Could you check a few things on this drawing? It's one solid part, dimensions in mm from its lowest x, y, z. A direction names the side the tool comes from. Round coordinates to 2 decimals unless told otherwise and drop trailing zeros. Loops run counter-clockwise (first coordinate to the right, second up) from the corner with the lowest first, then second, coordinate; pieces in that order, holes last.
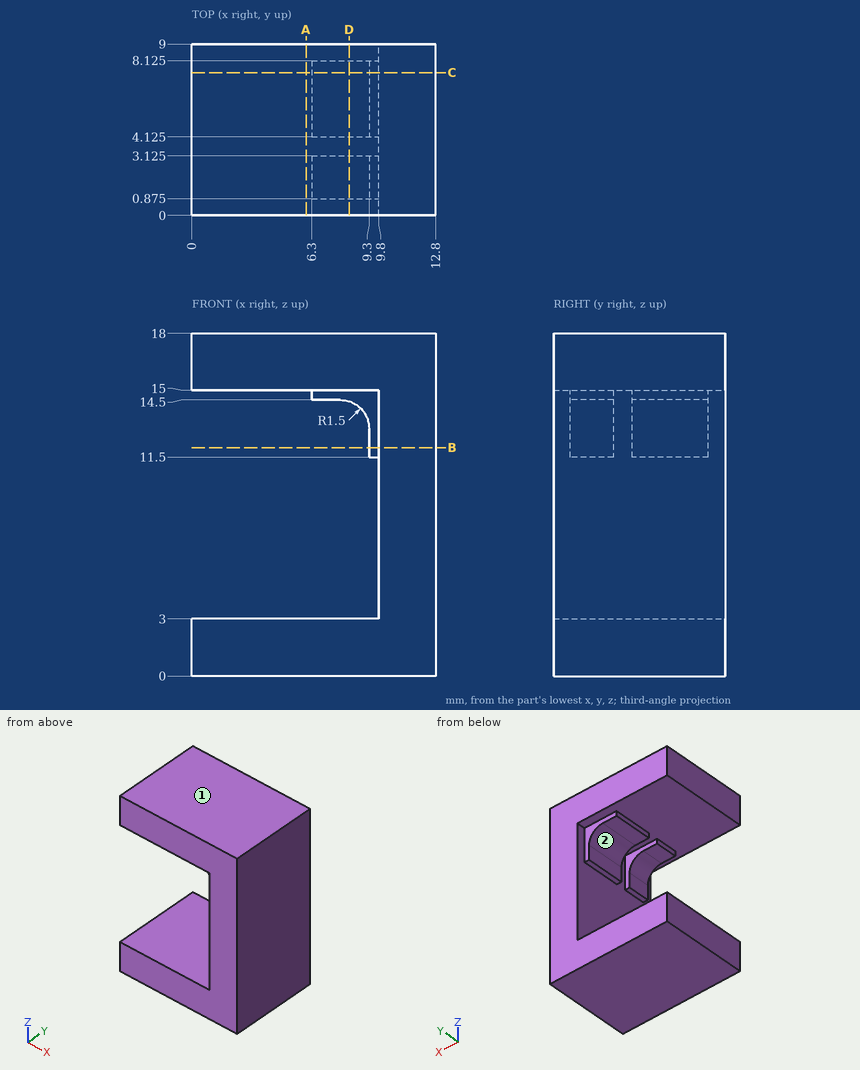
(1) If I drill on line 1 (Z direction, x = 1.75, y = 1.75); line 2 (Z direction, x = 6.5, y = 4.25); line 3 (X direction, y = 5.5, z = 12.5), over which ranges is the centre line in solid material (lowest first)?
(2) Suppose I cut it at D-D (x = 8.25). Write out the boundary of the cut face in (y, z) (3 decimals).
(3) Suppose I cut it at C-C (y = 7.5). Write out the boundary of the cut face in (x, z).
(4) Suppose I cut it at A-A (x = 6). Write out the boundary of the cut face in (y, z), then the cut area to 3 significant figures.
(5) Which directions (+Z, -Z, +X, -X, +Y, -Y) give clear straight access to the entire face, cutting with the end or side of a thin tool? Please do the marked faces 1 and 2.
(6) Suppose I cut it at B-B (z = 12). Write out the boundary of the cut face in (x, y) (3 decimals).
(7) For pin 1 (3 mm diameter, centred on x = 8.5, z = 13, fed in from -Y); pin 2 (1 mm diameter, centred on y = 7, z = 5.5, fed in from -X); pin 3 (3 mm diameter, centred on x = 7.5, z = 12.5, fed in from +Y); pin 4 (1.6 mm diameter, centred on y = 7, z = 12, fed in from -X), each with a flat end and sliding along its axis, tell me the tip position at first contact or that it passes through.
Check result:
1. line 1: z = 0 to 3, 15 to 18
1. line 2: z = 0 to 3, 14.5 to 18
1. line 3: x = 9.3 to 12.8
2. outline: (0, 0) - (9, 0) - (9, 3) - (0, 3) - close; (0, 15) - (0.875, 15) - (0.875, 14.431) - (3.125, 14.431) - (3.125, 15) - (4.125, 15) - (4.125, 14.431) - (8.125, 14.431) - (8.125, 15) - (9, 15) - (9, 18) - (0, 18) - close
3. outline: (0, 0) - (12.8, 0) - (12.8, 18) - (0, 18) - (0, 15) - (6.3, 15) - (6.3, 14.5) - (7.8, 14.5) arc R1.5 cw to (9.3, 13) - (9.3, 11.5) - (9.8, 11.5) - (9.8, 3) - (0, 3) - close
4. outline: (0, 0) - (9, 0) - (9, 3) - (0, 3) - close; (0, 15) - (9, 15) - (9, 18) - (0, 18) - close
4. area: 54.0 mm2
5. face 1: +Z, +X, -X, +Y, -Y
5. face 2: -X, +Y, -Y
6. outline: (9.3, 0.875) - (9.8, 0.875) - (9.8, 0) - (12.8, 0) - (12.8, 9) - (9.8, 9) - (9.8, 8.125) - (9.3, 8.125) - (9.3, 4.125) - (9.8, 4.125) - (9.8, 3.125) - (9.3, 3.125) - close
7. pin 1: stops at y = 0
7. pin 2: stops at x = 9.8
7. pin 3: passes through
7. pin 4: stops at x = 9.3
